For this review, take the finished solid that the model builds, in its own axes (mm). Coordinates: 2 decimals unless noted, no trailing zeros. Write each loop counter-clockwise with the first axis right and the second up, starting at its lowest first coordinate (ties: lowest second). Pieces come first, ordered by that corner, then holes.
```python
from build123d import *

# Parameters (mm, degrees)
SKETCH1_W           = 64
SKETCH1_H           = 11
BOSS_EXTRUDE1_DEPTH = 7
SKETCH3_R           = 1.7
CUT_EXTRUDE1_DEPTH  = 66.314623171


with BuildPart() as part:
    # Sketch1 → Boss-Extrude1 (new body)
    with BuildSketch(Plane.XY):
        with Locations((32, 5.5)):
            Rectangle(SKETCH1_W, SKETCH1_H)
    extrude(amount=-BOSS_EXTRUDE1_DEPTH)

    # Sketch3 → Cut-Extrude1 (cut, through all)
    with BuildSketch(Plane.XY):
        with Locations((6, 5.5)):
            Circle(SKETCH3_R)
        with Locations((58, 5.5)):
            Circle(SKETCH3_R)
    extrude(amount=-CUT_EXTRUDE1_DEPTH, mode=Mode.SUBTRACT)

    # Sketch7 → Cut-Revolve1 (revolve, cut)
    with BuildSketch(Plane(origin=(0, 5.5, 0), x_dir=(1, 0, 0), z_dir=(0, 1, 0)), mode=Mode.PRIVATE) as cut_revolve1_sk:
        Polygon((3.25, 0), (6, 0), (6, 2.75), align=None)
    cut_revolve1 = revolve(cut_revolve1_sk.sketch.rotate(Axis((6, 5.5, -2.75), (0, 0, 1)), 180), axis=Axis((6, 5.5, -2.75), (0, 0, 1)), mode=Mode.SUBTRACT)

    # Mirror1: Cut-Revolve1 across plane
    add(cut_revolve1.mirror(Plane(origin=(32, 0, 0), x_dir=(0, 0, 1), z_dir=(1, 0, 0))), mode=Mode.SUBTRACT)


solid = part.part
```
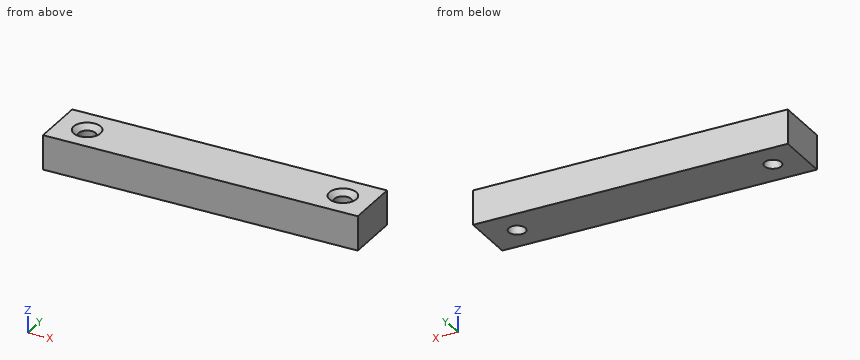
Q1. Add section C-C (z = -2). State the section outline as (x, y) points.
Ans:
outline: (0, 0) - (64, 0) - (64, 11) - (0, 11) - close; hole circle Ø3.4 at (6, 5.5); hole circle Ø3.4 at (58, 5.5)
Q2. For probe 1 along Y at (x, z) = (6, -3.2); probe 2 along X at (y, z) = (4.25, -5); probe 3 along Y at (x, z) = (56.5, -4), list the stretches that pass through material, from the lowest coordinate up.
Ans:
probe 1: y = 0 to 3.8, 7.2 to 11
probe 2: x = 0 to 4.85, 7.15 to 56.85, 59.15 to 64
probe 3: y = 0 to 4.7, 6.3 to 11
Q3. Add section B-B (x = 6). State the section outline as (y, z) points.
Ans:
outline: (0, -7) - (3.8, -7) - (3.8, -1.05) - (2.75, 0) - (0, 0) - close; (7.2, -7) - (11, -7) - (11, 0) - (8.25, 0) - (7.2, -1.05) - close
Q4. Add section A-A (y = 5.5). State the section outline as (x, z) points, then the cut area to 3 significant figures.
Ans:
outline: (0, -7) - (4.3, -7) - (4.3, -1.05) - (3.25, 0) - (0, 0) - close; (7.7, -7) - (56.3, -7) - (56.3, -1.05) - (55.25, 0) - (8.75, 0) - (7.7, -1.05) - close; (59.7, -7) - (64, -7) - (64, 0) - (60.75, 0) - (59.7, -1.05) - close
area: 398 mm2
Q5. Clearance check with flat-ended pins moving along their axes: pin 1 Ø2 at (x, y) = (52.5, 7) entering from +Z; pin 2 Ø4.5 at (x, y) = (6, 5.5) entering from +Z. State where each tip first meets the part, or that it passes through.
Ans:
pin 1: stops at z = 0
pin 2: stops at z = -0.5
